Input: part model. Units: mm. Frame: model coordinates. Face numbers are marked on the shaded views. Coordinates: 2 decimals unless noted, no trailing zeros. Write each loop counter-clockwise with the first axis right and the second up, starting at its lowest first coordinate (ties: lowest second). Pieces come first, ordered by that corner, then holes.
1) Section query B-B (z = 0). Output: boundary loops of the cut face in (x, y) (3 decimals), then the cut area to 3 significant figures.
2) Line query: L1, parallel to X at y = 2.5, z = 0 (3 decimals); L2, parallel to X at y = 10.45, z = 0 (3 decimals); L3, parallel to Z at x = 21, y = 5.25 (3 decimals). Output: solid intervals per line, ascending.
3) Section query A-A (x = -19.05). Output: boundary loops of the cut face in (y, z) (3 decimals).
4) Section query C-C (y = 8.5). Output: boundary loops of the cut face in (x, z) (3 decimals), then the cut area to 3 significant figures.
5) Draft query along X for the marked faces 1, 2, 3 and 4. Return one class per face: pulls with the +X half, pulls with the -X half, needs draft (parallel to the pull), parting line crosses it, or undercut.
6) Pin query (flat end, axial travel): pin 1 Ø8.5 at (x, z) = (-19.05, 0) entering from +Y; pin 2 Ø6 at (x, z) = (19.05, 0) entering from +Y. Return the tip coordinate at first contact, or that it passes through.
7) Section query D-D (x = 19.05). Output: boundary loops of the cut face in (y, z) (3 decimals), then the cut area to 3 significant figures.
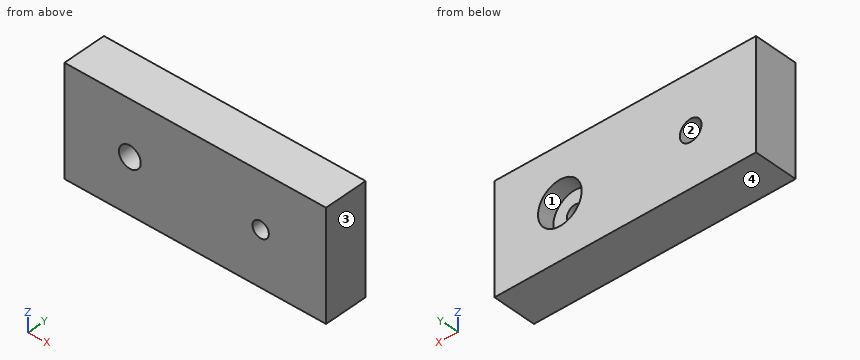
from build123d import *

# Parameters (mm, degrees)
SKETCH1_W           = 76.2
SKETCH1_H           = 31.75
BOSS_EXTRUDE1_DEPTH = 12.7
SKETCH2_R           = 3.175
SKETCH2_R_2         = 2.38125
CUT_EXTRUDE1_DEPTH  = 44.184668865
SKETCH3_R           = 6.35
CUT_EXTRUDE2_DEPTH  = 4.9022


with BuildPart() as part:
    # Sketch1 → Boss-Extrude1 (new body)
    with BuildSketch(Plane(origin=(0, 0, 0), x_dir=(1, 0, 0), z_dir=(0, 1, 0))):
        Rectangle(SKETCH1_W, SKETCH1_H)
    extrude(amount=BOSS_EXTRUDE1_DEPTH)

    # Sketch2 → Cut-Extrude1 (cut, through all)
    with BuildSketch(Plane(origin=(0, 12.7, 0), x_dir=(1, 0, 0), z_dir=(0, 1, 0))):
        with Locations(Location((-19.05, 0, 0), (0, 0, 270))):
            Circle(SKETCH2_R)
        with Locations(Location((19.05, 0, 0), (0, 0, 270))):
            Circle(SKETCH2_R_2)
    extrude(amount=-CUT_EXTRUDE1_DEPTH, mode=Mode.SUBTRACT)

    # Sketch3 → Cut-Extrude2 (cut)
    with BuildSketch(Plane(origin=(0, 12.7, 0), x_dir=(1, 0, 0), z_dir=(0, 1, 0))):
        with Locations(Location((19.05, 0, 0), (0, 0, 270))):
            Circle(SKETCH3_R)
    extrude(amount=-CUT_EXTRUDE2_DEPTH, mode=Mode.SUBTRACT)


solid = part.part
Answer:
1. outline: (-38.1, 0) - (-22.225, 0) - (-22.225, 12.7) - (-38.1, 12.7) - close; (-15.875, 0) - (16.669, 0) - (16.669, 7.798) - (12.7, 7.798) - (12.7, 12.7) - (-15.875, 12.7) - close; (21.431, 0) - (38.1, 0) - (38.1, 12.7) - (25.4, 12.7) - (25.4, 7.798) - (21.431, 7.798) - close
1. area: 788 mm2
2. L1: x = -38.1 to -22.225, -15.875 to 16.669, 21.431 to 38.1
2. L2: x = -38.1 to -22.225, -15.875 to 12.7, 25.4 to 38.1
2. L3: z = -15.875 to -1.367, 1.367 to 15.875
3. outline: (0, -15.875) - (12.7, -15.875) - (12.7, -3.175) - (0, -3.175) - close; (0, 3.175) - (12.7, 3.175) - (12.7, 15.875) - (0, 15.875) - close
4. outline: (-38.1, -15.875) - (38.1, -15.875) - (38.1, 15.875) - (-38.1, 15.875) - close; hole circle Ø6.35 at (-19.05, 0); hole circle Ø12.7 at (19.05, 0)
4. area: 2,260 mm2
5. face 1: undercut
5. face 2: undercut
5. face 3: pulls with the +X half
5. face 4: needs draft
6. pin 1: stops at y = 12.7
6. pin 2: stops at y = 7.8
7. outline: (0, -15.875) - (12.7, -15.875) - (12.7, -6.35) - (7.798, -6.35) - (7.798, -2.381) - (0, -2.381) - close; (0, 2.381) - (7.798, 2.381) - (7.798, 6.35) - (12.7, 6.35) - (12.7, 15.875) - (0, 15.875) - close
7. area: 304 mm2
